Could you check a few things on this model? Use its own coordinates, in mm. Face numbers are marked on the shaded views. A direction names the side the tool comes from. Round coordinates to 2 decimals unless told otherwise and drop trailing zeros. Order: outer loops, then holes, each group sorted by start corner. A loop starts at its lowest first (then second) coordinate and runs counter-clockwise, first axis right, second up. Notation, with made-up numbers: (85, 6) - (116, 6) arc R21 cw to (116, 42) - close; hole circle Ø8 at (79, -12.75). An arc over 180 degrees is marked (long way). Return JSON: item names as keys, results as strings. Group by question number.
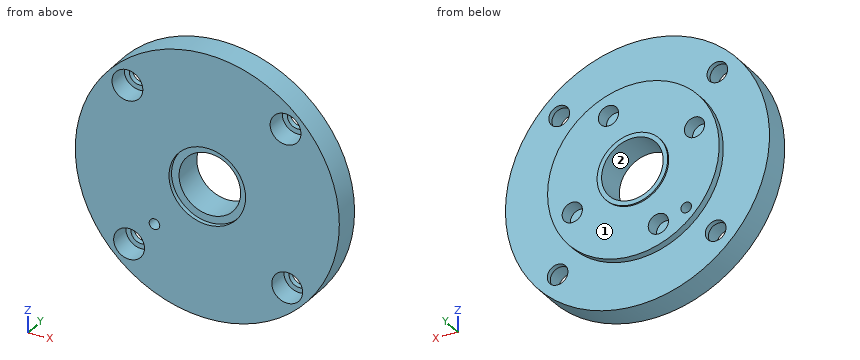
from build123d import *

# Parameters (mm, degrees)
IZIM1_R                     = 150
Y_KSEKLIK_EKSTR_ZYON1_DEPTH = 30
IZIM2_R                     = 97.5
Y_KSEKLIK_EKSTR_ZYON2_DEPTH = 8
IZIM3_R                     = 40.15
Y_KSEKLIK_EKSTR_ZYON3_DEPTH = 2
IZIM4_R                     = 35
KES_EKSTR_ZYON1_DEPTH       = 41
IZIM5_R                     = 43.5
KES_EKSTR_ZYON2_DEPTH       = 5
IZIM6_R                     = 11.5
IZIM6_R_2                   = 6
KES_EKSTR_ZYON4_DEPTH       = 16
IZIM7_R                     = 11.75
KES_EKSTR_ZYON5_DEPTH       = 31
IZIM8_R                     = 6
KES_EKSTR_ZYON6_DEPTH       = 23
IZIM9_R                     = 17.5
KES_EKSTR_ZYON7_DEPTH       = 24


with BuildPart() as part:
    # Çizim1 → Yükseklik-Ekstrüzyon1 (new body)
    with BuildSketch(Plane(origin=(0, 0, 0), x_dir=(1, 0, 0), z_dir=(0, 1, 0))):
        Circle(IZIM1_R)
    extrude(amount=Y_KSEKLIK_EKSTR_ZYON1_DEPTH)

    # Çizim2 → Yükseklik-Ekstrüzyon2 (add)
    with BuildSketch(Plane(origin=(0, 30, 0), x_dir=(1, 0, 0), z_dir=(0, 1, 0))):
        Circle(IZIM2_R)
    extrude(amount=Y_KSEKLIK_EKSTR_ZYON2_DEPTH)

    # Çizim3 → Yükseklik-Ekstrüzyon3 (add)
    with BuildSketch(Plane(origin=(0, 38, 0), x_dir=(1, 0, 0), z_dir=(0, 1, 0))):
        Circle(IZIM3_R)
    extrude(amount=Y_KSEKLIK_EKSTR_ZYON3_DEPTH)

    # Çizim4 → Kes-Ekstrüzyon1 (cut, through all)
    with BuildSketch(Plane(origin=(0, 40, 0), x_dir=(1, 0, 0), z_dir=(0, 1, 0))):
        Circle(IZIM4_R)
    extrude(amount=-KES_EKSTR_ZYON1_DEPTH, mode=Mode.SUBTRACT)

    # Çizim5 → Kes-Ekstrüzyon2 (cut)
    with BuildSketch(Plane.XZ):
        Circle(IZIM5_R)
    extrude(amount=-KES_EKSTR_ZYON2_DEPTH, mode=Mode.SUBTRACT)

    # Çizim6 → Kes-Ekstrüzyon4 (cut)
    with BuildSketch(Plane(origin=(0, 38, 0), x_dir=(1, 0, 0), z_dir=(0, 1, 0))):
        with Locations((-28.338059011, 69.440293861)):
            Circle(IZIM6_R)
        with Locations((69.440293861, 28.338059011)):
            Circle(IZIM6_R)
        with Locations((28.338059011, -69.440293861)):
            Circle(IZIM6_R)
        with Locations((-69.440293861, -28.338059011)):
            Circle(IZIM6_R)
        with Locations((-60, 60)):
            Circle(IZIM6_R_2)
    extrude(amount=-KES_EKSTR_ZYON4_DEPTH, mode=Mode.SUBTRACT)

    # Çizim7 → Kes-Ekstrüzyon5 (cut, through all)
    with BuildSketch(Plane(origin=(0, 30, 0), x_dir=(1, 0, 0), z_dir=(0, 1, 0))):
        with Locations((-88.857244245, 90.738030313)):
            Circle(IZIM7_R)
        with Locations((90.738030313, 88.857244245)):
            Circle(IZIM7_R)
        with Locations((88.857244245, -90.738030313)):
            Circle(IZIM7_R)
        with Locations((-90.738030313, -88.857244245)):
            Circle(IZIM7_R)
    extrude(amount=-KES_EKSTR_ZYON5_DEPTH, mode=Mode.SUBTRACT)

    # Çizim8 → Kes-Ekstrüzyon6 (cut, through all)
    with BuildSketch(Plane(origin=(0, 22, 0), x_dir=(1, 0, 0), z_dir=(0, 1, 0))):
        with Locations((-60, 60)):
            Circle(IZIM8_R)
    extrude(amount=-KES_EKSTR_ZYON6_DEPTH, mode=Mode.SUBTRACT)

    # Çizim9 → Kes-Ekstrüzyon7 (cut)
    with BuildSketch(Plane.XZ):
        with Locations((-90.738030313, 88.857244245)):
            Circle(IZIM9_R)
        with Locations((88.857244245, 90.738030313)):
            Circle(IZIM9_R)
        with Locations((90.738030313, -88.857244245)):
            Circle(IZIM9_R)
        with Locations((-88.857244245, -90.738030313)):
            Circle(IZIM9_R)
    extrude(amount=-KES_EKSTR_ZYON7_DEPTH, mode=Mode.SUBTRACT)


solid = part.part
1) For the marked faces 1 and 2, which set-ups out of +Z, -Z, +X, -X, +Y, -Y let a thin tool reach every point of the face, with its end or its side?
2) I want a section at C-C, the plane y = 33.5. List the corners of the cut face in (x, z) for me, plus the area to 3 significant figures.
3) I want a section at B-B, the plane z = 0. List the corners of the cut face in (x, y) for me.
4) If I drill on line 1 along Z through (x, y) = (-31.5, 30.5); line 2 along X through (y, z) = (34, -59); line 3 along Y through (x, z) = (27, -80), over which ranges is the centre line in solid material (lowest first)? Write a range as from..to.
5) I want a section at D-D, the plane y = 16. List the corners of the cut face in (x, z) for me, plus the area to 3 significant figures.
6) Will these pins go through, and if not, where does the flat tip stop? pin 1 (12 mm diameter, centred on x = -106, y = 25.5, fed in from -Z); pin 2 (10 mm diameter, centred on y = 34.5, z = -64.5, fed in from +X); pin 3 (17.5 mm diameter, centred on x = -93.5, z = 93.5, fed in from -Y); pin 4 (14 mm diameter, centred on x = 90.74, z = -88.86, fed in from +Y).
7) I want a section at A-A, the plane x = 0. List the corners of the cut face in (y, z) for me.
Outcome:
{
 "1": {"face 1": "+Y", "face 2": "+Y, -Y"},
 "2": {"outline": "circle Ø195 at (0, 0); hole circle Ø23 at (-69.44, 28.34); hole circle Ø12 at (-60, -60); hole circle Ø23 at (-28.34, -69.44); hole circle Ø70 at (0, 0); hole circle Ø23 at (28.34, 69.44); hole circle Ø23 at (69.44, -28.34)", "area": "24,200 mm^2"},
 "3": {"outline": "(-150, 0) - (-43.5, 0) - (-43.5, 5) - (-35, 5) - (-35, 40) - (-40.15, 40) - (-40.15, 38) - (-97.5, 38) - (-97.5, 30) - (-150, 30) - close; (35, 5) - (43.5, 5) - (43.5, 0) - (150, 0) - (150, 30) - (97.5, 30) - (97.5, 38) - (40.15, 38) - (40.15, 40) - (35, 40) - close"},
 "4": {"line 1": "-92.27..-80.5, -58.38..-15.26, 15.26..92.27", "line 2": "-77.62..-65.92, -54.08..-33.16, -23.52..77.62", "line 3": "0..38"},
 "5": {"outline": "circle Ø300 at (0, 0); hole circle Ø35 at (-90.74, 88.86); hole circle Ø35 at (-88.86, -90.74); hole circle Ø12 at (-60, -60); hole circle Ø70 at (0, 0); hole circle Ø35 at (88.86, 90.74); hole circle Ø35 at (90.74, -88.86)", "area": "62,900 mm^2"},
 "6": {"pin 1": "z = -111.8", "pin 2": "x = 136.44", "pin 3": "y = 24", "pin 4": "through"},
 "7": {"outline": "(0, -150) - (30, -150) - (30, -97.5) - (38, -97.5) - (38, -40.15) - (40, -40.15) - (40, -35) - (5, -35) - (5, -43.5) - (0, -43.5) - close; (0, 43.5) - (5, 43.5) - (5, 35) - (40, 35) - (40, 40.15) - (38, 40.15) - (38, 97.5) - (30, 97.5) - (30, 150) - (0, 150) - close"}
}
